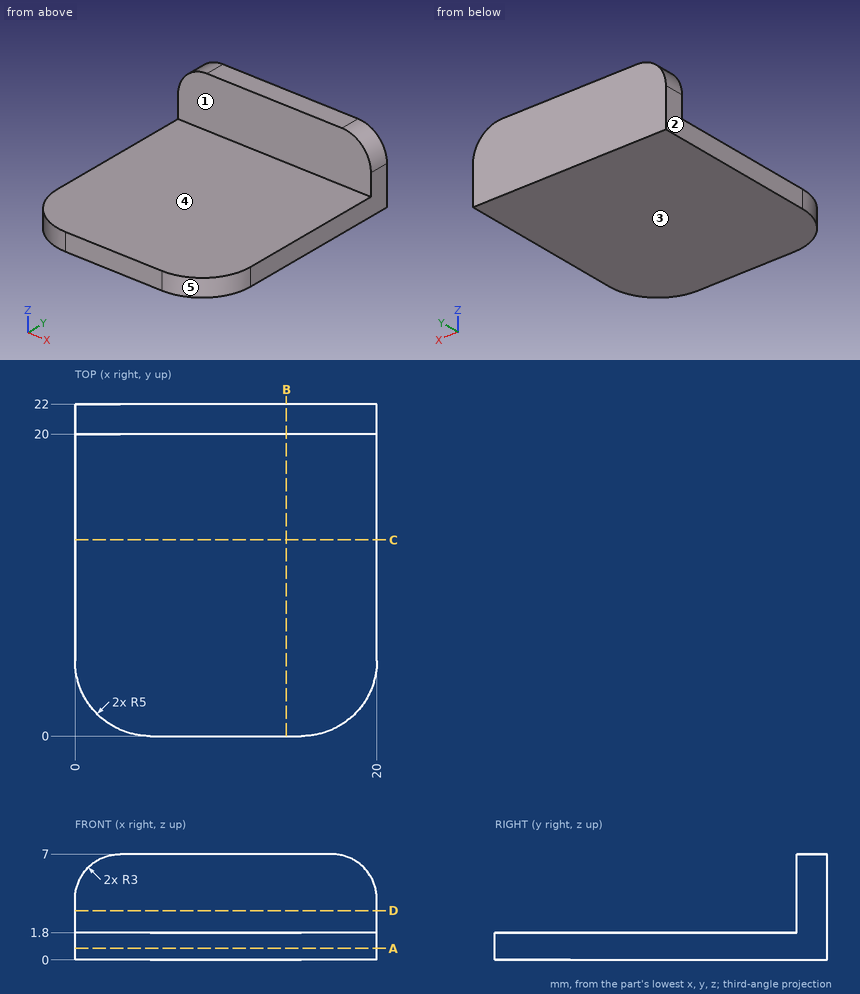
Print and shaded views of the part. All mm, measured from the part's lowest x, y and z. A direction names the side the tool comes from. Give positions to 0.01 mm unless a question says otherwise; leave off trailing zeros. Loops run counter-clockwise (first coordinate to the right, second up) from the corner with the lowest first, then second, coordinate; pieces in that order, holes last. Notation, with made-up numbers: (-8, -14.75) -> (48, -14.75) arc R17 cw to (48, 7.25) -> close; hole circle Ø9 at (-35, -39.5). An arc over 180 degrees is marked (long way). Use a Markdown table: item, result.
1. Mould opens along Z. For the marked faces 3, 4 and 5 say: pulls with the +Z half, pulls with the -Z half, needs draft (parallel to the pull), parting line crosses it, or undercut.
Check result:
| item | result |
|---|---|
| face 3 | pulls with the -Z half |
| face 4 | pulls with the +Z half |
| face 5 | needs draft |
2. Flat gauge pins, fed straight in: pin 1 (4 mm diameter, centred on x = 9.5, z = 5.5, fed in from -Y); pin 2 (10 mm diameter, centred on x = 9, y = 13.5, fed in from +Z). Where does each tip first touch, or does it go through?
Check result:
| item | result |
|---|---|
| pin 1 | stops at y = 20 |
| pin 2 | stops at z = 1.8 |
3. Wall check: L1, parallel to Z at x = 7, y = 15.75; L2, parallel to Y at x = 13.25, z = 5; L3, parallel to X at y = 1, z = 0.5. Give the ranges that are in metal, low to high. Write a range as [from, to].
Check result:
| item | result |
|---|---|
| L1 | z = [0, 1.8] |
| L2 | y = [20, 22] |
| L3 | x = [2, 18] |
4. Slice it at C-C (y = 13). List the corners of the cut face in (x, z).
Check result:
| item | result |
|---|---|
| outline | (0, 0) -> (20, 0) -> (20, 1.8) -> (0, 1.8) -> close |
5. Slice it at B-B (x = 14). List the corners of the cut face in (y, z), plus the area to 3 significant figures.
Check result:
| item | result |
|---|---|
| outline | (0, 0) -> (22, 0) -> (22, 7) -> (20, 7) -> (20, 1.8) -> (0, 1.8) -> close |
| area | 50.0 mm^2 |
6. Slice it at D-D (z = 3.25). List the corners of the cut face in (x, y), plus the area to 3 significant figures.
Check result:
| item | result |
|---|---|
| outline | (0, 20) -> (20, 20) -> (20, 22) -> (0, 22) -> close |
| area | 40.0 mm^2 |
7. Slice it at A-A (z = 0.75). List the corners of the cut face in (x, y).
Check result:
| item | result |
|---|---|
| outline | (0, 5) arc R5 ccw to (5, 0) -> (15, 0) arc R5 ccw to (20, 5) -> (20, 22) -> (0, 22) -> close |
8. Which spindle directions (+Z, -Z, +X, -X, +Y, -Y) get a long thin tool onto all of the face, cutting with end or side? Do the marked faces 1 and 2. Say none if no direction does.
Check result:
| item | result |
|---|---|
| face 1 | +Z, +X, -X, -Y |
| face 2 | +Z, -Z, -X, +Y, -Y |
